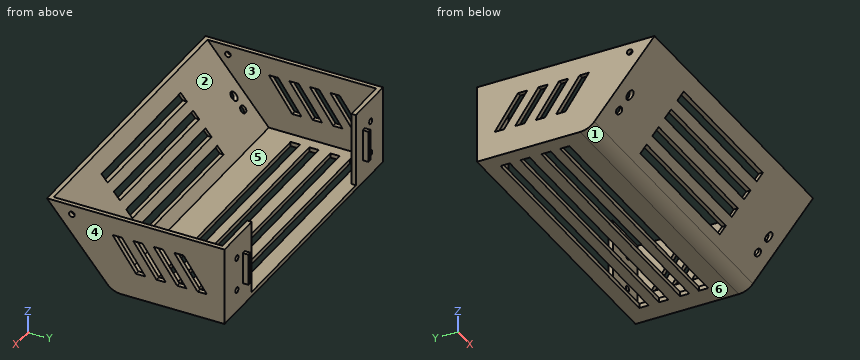
Autodesk Inventor part; units mm, degrees
ref_plane "Work Plane1" through (0, -50, 0) normal (0, 1, 0) x (-1, 0, 0)
ref_plane "YZ Plane" through (0, 0, 0) normal (1, 0, 0) x (0, 1, 0)
ref_plane "XY Plane" through (0, 0, 0) normal (0, 0, 1) x (1, 0, 0)
sketch "Sketch1" plane through (0, 0, 0) normal (0, 0, 1) x (1, 0, 0)
  line L0 (0, 0) -> (160, 0)
  line L1 (160, 0) -> (160, 60)
  line L2 (160, 60) -> (0, 60)
  line L3 (0, 60) -> (0, 0)
  line L4 (8.5291, 51.8697) -> (148.5291, 51.8697)
  line L5 (148.5291, 51.8697) -> (148.5291, 46.8697)
  line L6 (148.5291, 46.8697) -> (8.5291, 46.8697)
  line L7 (8.5291, 46.8697) -> (8.5291, 51.8697)
  line L8 (8.5291, 41.2311) -> (148.5291, 41.2311)
  line L9 (148.5291, 41.2311) -> (148.5291, 36.2311)
  line L10 (148.5291, 36.2311) -> (8.5291, 36.2311)
  line L11 (8.5291, 36.2311) -> (8.5291, 41.2311)
  line L12 (8.5291, 30) -> (148.5291, 30)
  line L13 (148.5291, 30) -> (148.5291, 25)
  line L14 (148.5291, 25) -> (8.5291, 25)
  line L15 (8.5291, 25) -> (8.5291, 30)
  line L16 (8.5291, 19.9539) -> (148.5291, 19.9539)
  line L17 (148.5291, 19.9539) -> (148.5291, 14.9539)
  line L18 (148.5291, 14.9539) -> (8.5291, 14.9539)
  line L19 (8.5291, 14.9539) -> (8.5291, 19.9539)
  dimension "d0" = 160
  dimension "d1" = 60
  dimension "d2" = 140
  dimension "d3" = 5
  dimension "d4" = 5
  dimension "d5" = 5
  dimension "d6" = 5
extrude "Extrusion1" add sketch "Sketch1" along normal blind 2.4
sketch "Sketch2" plane through (0, 0, 2.4) normal (0, 0, 1) x (1, 0, 0)
  line L0 (0, 60) -> (0, 0)
  line L1 (0, 0) -> (160, 0)
  line L2 (0, 60) -> (2.4, 60)
  line L3 (2.4, 60) -> (2.4, 0)
  line L4 (2.4, 0) -> (0, 0)
  line L5 (0, 0) -> (0, 60)
  line L6 (160, 60) -> (0, 60)
  line L7 (160, 0) -> (157.6, 0)
  line L8 (157.6, 0) -> (157.6, 60)
  line L9 (157.6, 60) -> (160, 60)
  line L10 (160, 60) -> (160, 0)
  dimension "d9" = 2.4
  dimension "d10" = 2.4
extrude "Extrusion2" add sketch "Sketch2" along normal blind 39.6 contours L2 L3 L1 L0 | L6 L10 L1 L8
sketch "Sketch3" plane through (160, 0, 0) normal (1, 0, 0) x (0, 0, -1)
  line L0 (0, 0) -> (-42, -35.2422)
  line L1 (0, 0) -> (54.8271, 0) construction
  line L2 (-42, 0) -> (-42, 60)
  line L3 (-42, -35.2422) -> (-42, 0)
  line L4 (-42, 0) -> (0, 0)
  dimension "d13" = 140
extrude "Extrusion3" add sketch "Sketch3" against normal blind 2.4
sketch "Sketch4" plane through (0, 0, 0) normal (-1, 0, 0) x (0, 0, 1)
  line L0 (0, 0) -> (42, 0)
  line L1 (42, 0) -> (0, 0)
  line L2 (0, 0) -> (42, -35.2422)
  line L3 (0, 0) -> (42, -35.2422)
  line L4 (42, -35.2422) -> (42, 0)
extrude "Extrusion4" add sketch "Sketch4" against normal blind 2.4
sketch "Sketch5" plane through (157.6, 0, 2.4) normal (-1, 0, 0) x (0, 0, 1)
  line L0 (-2.4, 0) -> (0, 0)
  line L1 (39.6, 60) -> (39.6, -35.2422)
  line L2 (39.6, -35.2422) -> (39.6, -32.8422)
  line L3 (39.6, -32.8422) -> (0, 0)
  line L4 (-2.4, 0) -> (39.6, -35.2422)
  dimension "d18" = 2.4
extrude "Extrusion5" add sketch "Sketch5" along normal blind 157.6
sketch "Sketch6" plane through (160, 60, 42) normal (1, 0, 0) x (0, 0, -1)
  line L0 (10, -60) -> (10, -55)
  line L1 (10, -49) -> (10, -44)
  line L2 (10, -38) -> (10, -33)
  line L3 (10, -27) -> (10, -22)
  line L4 (10, -22) -> (28.0953, -9.4875)
  line L5 (28.0953, -9.4875) -> (28.0953, -14.4875)
  line L6 (42, 0) -> (0, 0)
  line L7 (28.0953, -20.4875) -> (28.0953, -25.4875)
  line L8 (28.0953, -31.4875) -> (28.0953, -36.4875)
  line L9 (28.0953, -42.4875) -> (28.0953, -47.4875)
  line L10 (28.0953, -47.4875) -> (10, -60)
  line L11 (28.0953, -42.4875) -> (10, -55)
  line L12 (28.0953, -36.4875) -> (10, -49)
  line L13 (10, -44) -> (28.0953, -31.4875)
  line L14 (28.0953, -25.4875) -> (10, -38)
  line L15 (10, -33) -> (28.0953, -20.4875)
  line L16 (28.0953, -14.4875) -> (10, -27)
  line L17 (0, -95.2422) -> (0, 0)
  circle A0 centre (5, -81.9088) radius 1.5
  line L18 (42, -60) -> (0, -95.2422)
  dimension "d21" = 5
  dimension "d22" = 6
  dimension "d23" = 5
  dimension "d24" = 6
  dimension "d25" = 5
  dimension "d26" = 6
  dimension "d27" = 5
  dimension "d28" = 22
  dimension "d29" = 5
  dimension "d30" = 6
  dimension "d31" = 5
  dimension "d32" = 6
  dimension "d33" = 5
  dimension "d34" = 6
  dimension "d35" = 5
  dimension "d36" = 10
  dimension "d77" = 3
  dimension "d78" = 7
  dimension "d79" = 5
ref_plane "Work Plane1" through (0, -50, 0) normal (0, 1, 0) x (-1, 0, 0)
sketch "Sketch7" plane through (0, -50, 0) normal (0, 1, 0) x (-1, 0, 0)
  circle A0 centre (-10, 20) radius 2
  line L0 (-157.6, 42) -> (-2.4, 42)
  line L1 (-80, 42) -> (-80, 0)
  line L2 (-8.5291, 0) -> (-148.5291, 0)
  circle A1 centre (-150, 20) radius 2
  line L3 (-160, 0) -> (-160, 42)
  line L4 (0, 0) -> (0, 42)
  line L5 (0, 0) -> (-160, 0)
  line L6 (-80, 35.2897) -> (-40, 35.2897)
  line L7 (-40, 35.2897) -> (-40, 31.2897)
  line L8 (-40, 31.2897) -> (-120, 31.2897)
  line L9 (-120, 31.2897) -> (-120, 35.2897)
  line L10 (-120, 35.2897) -> (-80, 35.2897)
  line L11 (-39.9996, 27.2897) -> (-39.9998, 23.2897)
  line L12 (-40, 19.2897) -> (-40, 15.2897)
  line L13 (-40, 15.2897) -> (-120, 15.2897)
  line L14 (-120, 15.2897) -> (-120, 19.2897)
  line L15 (-120, 19.2897) -> (-40, 19.2897)
  line L16 (-39.9998, 23.2897) -> (-120, 23.2897)
  line L17 (-120, 23.2897) -> (-120, 27.2897)
  line L18 (-120, 27.2897) -> (-39.9996, 27.2897)
  line L19 (-40.1762, 11.5108) -> (-40.1762, 7.5108)
  line L20 (-40.1762, 7.5108) -> (-120.1762, 7.5108)
  line L21 (-120.1762, 7.5108) -> (-120.1762, 11.5108)
  line L22 (-120.1762, 11.5108) -> (-40.1762, 11.5108)
  dimension "d40" = 4
  dimension "d41" = 4
  dimension "d42" = 10
  dimension "d43" = 10
  dimension "d44" = 20
  dimension "d45" = 20
  dimension "d46" = 40
  dimension "d47" = 4
  dimension "d49" = 4
  dimension "d50" = 4
  dimension "d51" = 4
  dimension "d52" = 4
  dimension "d55" = 4
  dimension "d56" = 80
  dimension "d57" = 80
  dimension "d58" = 80
  dimension "d59" = 80.0002
  dimension "d60" = 80
extrude "Extrusion8" cut sketch "Sketch7" along normal blind 160
sketch "Sketch8" plane through (0, -35.2422, 42) normal (0, -0.766, -0.6428) x (1, 0, 0)
  circle A0 centre (10, -37.8271) radius 2
  line L0 (0, -54.8271) -> (0, 0)
  circle A1 centre (150, -37.8271) radius 2
  line L1 (160, -54.8271) -> (160, 0)
  line L2 (0, -54.8271) -> (160, -54.8271)
  dimension "d63" = 4
  dimension "d64" = 10
  dimension "d65" = 4
  dimension "d66" = 10
  dimension "d67" = 17
  dimension "d68" = 17
extrude "Extrusion9" cut sketch "Sketch8" against normal blind 160
sketch "Sketch9" plane through (157.6, 60, 2.4) normal (-1, 0, 0) x (0, 0, 1)
  line L0 (39.6, 0) -> (39.6, -92.8422)
  line L1 (0, 0) -> (39.6, 0)
  line L2 (39.6, 0) -> (39.6, -2.4)
  line L3 (39.6, -2.4) -> (0, -2.4)
  line L4 (0, -2.4) -> (0, 0)
  point P0 (-2.4, -60)
  dimension "d71" = 2.4
extrude "Extrusion10" add sketch "Sketch9" along normal blind 25
sketch "Sketch10" plane through (2.4, 60, 42) normal (1, 0, 0) x (0, 0, -1)
  line L0 (39.6, 0) -> (0, 0)
  line L1 (0, 0) -> (0, -92.8422)
  line L2 (39.6, 0) -> (0, 0)
  line L3 (0, 0) -> (0, -2.4)
  line L4 (0, -2.4) -> (39.6, -2.4)
  line L5 (39.6, -2.4) -> (39.6, 0)
  point P0 (42, -60)
  dimension "d74" = 2.4
extrude "Extrusion11" add sketch "Sketch10" along normal blind 25
extrude "Extrusion12" cut sketch "Sketch6" against normal blind 160
sketch "Sketch11" plane through (0, 60, 0) normal (0, 1, 0) x (1, 0, 0)
  circle A0 centre (147.5, -30) radius 1.5
  line L0 (160, 0) -> (160, -42)
  line L1 (160, -42) -> (132.6, -42)
  circle A1 centre (147.5, -12) radius 1.5
  line L2 (160, 0) -> (0, 0)
  circle A2 centre (12.5, -30) radius 1.5
  circle A3 centre (12.5, -12) radius 1.5
  line L3 (0, 0) -> (0, -42)
  line L4 (0, -42) -> (27.4, -42)
  line L5 (141.6, -29.5) -> (139.6, -29.5)
  line L6 (139.6, -29.5) -> (139.6, -12.5)
  line L7 (139.6, -12.5) -> (141.6, -12.5)
  line L8 (141.6, -12.5) -> (141.6, -29.5)
  line L9 (132.6, -42) -> (132.6, -2.4)
  line L10 (20.4, -29.5) -> (18.4, -29.5)
  line L11 (18.4, -29.5) -> (18.4, -12.5)
  line L12 (18.4, -12.5) -> (20.4, -12.5)
  line L13 (20.4, -12.5) -> (20.4, -29.5)
  line L14 (27.4, -2.4) -> (27.4, -42)
  dimension "d82" = 3
  dimension "d83" = 12.5
  dimension "d84" = 12
  dimension "d85" = 3
  dimension "d86" = 12.5
  dimension "d87" = 12
  dimension "d88" = 3
  dimension "d89" = 3
  dimension "d90" = 12.5
  dimension "d91" = 12
  dimension "d92" = 12
  dimension "d93" = 12.5
  dimension "d96" = 7
  dimension "d97" = 2
  dimension "d98" = 12.5
  dimension "d99" = 12.5
  dimension "d101" = 2
  dimension "d103" = 7
  dimension "d104" = 12.5
  dimension "d107" = 12.5
extrude "Extrusion13" cut sketch "Sketch11" against normal blind 12 contours A0 | A1 | A2 | A3
extrude "Extrusion14" add sketch "Sketch11" along normal blind 3 contours L5 L6 L7 L8 | L10 L11 L12 L13
fillet "Fillet1" radius 10 1 edges at (80, 0, 0)
equation "\"d42\" = d43"
equation "\"d45\" = d44"
equation "\"d66\" = d64"
equation "\"d68\" = d67"
equation "\"d86\" = d83"
equation "\"d87\" = d84"
equation "\"d90\" = d86"
equation "\"d91\" = d87"
equation "\"d92\" = d84"
equation "\"d93\" = d83"
equation "\"d103\" = d96"
equation "\"d104\" = d99"
equation "\"d107\" = d98"
properties part number "Chassi_Front"
Verification items for the finished model (mm, model axes). Face numbers are marked on the shaded views. A direction names the side the tool comes from. Round coordinates to 2 decimals unless told otherwise and drop trailing zeros.
(1) Mould release check, pull along Y, two halves, no side actions. Record for the marked faces 1, 2, 3 and 4: pulls with the +Y half, pulls with the -Y half, needs draft (parallel to the pull), parting line crosses it, or undercut.
Returned:
face 1: pulls with the -Y half
face 2: undercut
face 3: undercut
face 4: needs draft
(2) Material ranges on line 1 (Z direction, x = 147.5, y = 59.4); line 2 (X direction, y = -14, z = 20); line 3 (X direction, y = 59, z = 12), recorded low to high.
Returned:
line 1: z = 0 to 10.5, 13.5 to 28.5, 31.5 to 42
line 2: x = 0 to 2.4, 157.6 to 160
line 3: x = 0 to 11, 14 to 27.4, 132.6 to 146, 149 to 160
(3) Access from +Z, -Z, +X, -X, +Y, -Y to the whole of each face (thin tool, end or side, straight path). Record for the marked faces 5 and 6.
Returned:
face 5: +Z
face 6: -Z, +X, -X, +Y, -Y
(4) Section check A-A (x = 44.5). Give the number of separate pieces and of enclosed holes in the cut face, plus the area to 3 significant figures.
Returned:
separate pieces: 9
enclosed holes: 0
area: 148 mm2
(5) Depth check by flat-ended pin: pin 1 Ø1 at (x, z) = (115, 5) entering from -Y; pin 2 Ø1.2 at (x, z) = (85.5, 1.5) entering from +Y; pin 3 Ø6 at (y, z) = (-17.5, 14) entering from +X; pin 4 Ø1.2 at (y, z) = (28, 1.5) entering from -X. Enter the tip coordinate at first touch or a pass-through.
Returned:
pin 1: stops at y = -4.62
pin 2: stops at y = 60
pin 3: passes through
pin 4: stops at x = 0
